from build123d import *

# Parameters (mm, degrees)
ESQUISSE1_W                  = 210
ESQUISSE1_H                  = 90
ESQUISSE1_W_2                = 200
ESQUISSE1_H_2                = 80
BOSS_EXTRU_1_DEPTH           = 5
ESQUISSE2_R                  = 20
ESQUISSE2_R_2                = 15
BOSS_EXTRU_2_DEPTH           = 5
BOSS_EXTRU_3_DEPTH           = 90
BOSS_EXTRU_4_DEPTH           = 200
ESQUISSE6_W                  = 26.875595252
ESQUISSE6_H                  = 32.252188949
ENL_V_MAT_EXTRU_1_DEPTH      = 200
ENL_V_MAT_EXTRU_2_DEPTH      = 200
ENL_V_MAT_EXTRU_3_DEPTH      = 237
ESQUISSE10_R                 = 20
ENL_V_MAT_EXTRU_4_DEPTH      = 6
ENL_V_MAT_EXTRU_4_DEPTH_BACK = 106
ESQUISSE11_W                 = 294.385058415
ESQUISSE11_H                 = 160.265549893
ENL_V_MAT_EXTRU_5_DEPTH      = 23
ENL_V_MAT_EXTRU_5_DEPTH_BACK = 16
BOSS_EXTRU_5_DEPTH           = 5


with BuildPart() as part:
    # Esquisse1 → Boss.-Extru.1 (new body)
    with BuildSketch(Plane.XY):
        with Locations((100, -26.819835627)):
            Rectangle(ESQUISSE1_W, ESQUISSE1_H)
        with Locations((100, -26.819835627)):
            Rectangle(ESQUISSE1_W_2, ESQUISSE1_H_2, mode=Mode.SUBTRACT)
    extrude(amount=BOSS_EXTRU_1_DEPTH)



with BuildPart() as body_2:
    # Esquisse2 → Boss.-Extru.2 (new body)
    with BuildSketch(Plane.XY.offset(105)):
        with Locations((100, -26.819835627)):
            Circle(ESQUISSE2_R)
        with Locations((100, -26.819835627)):
            Circle(ESQUISSE2_R_2, mode=Mode.SUBTRACT)
    extrude(amount=BOSS_EXTRU_2_DEPTH)


with BuildPart() as part_1:
    add(part.part)

    add(body_2.part)  # Boss.-Extru.3 merges body 2
    # Esquisse3 → Boss.-Extru.3 (add)
    with BuildSketch(Plane.XZ.offset(71.819835627)):
        Polygon((113.437797626, 105), (198.437797626, 5), (205, 5), (119.954563332, 105), align=None)
        Polygon((80, 105), (-5, 5), (1.562202374, 5), (86.562202374, 105), align=None)
    extrude(amount=-BOSS_EXTRU_3_DEPTH)

    # Esquisse5 → Boss.-Extru.4 (add)
    with BuildSketch(Plane.ZY.offset(-200)):
        Polygon((5, 18.180164373), (105, -5.554833167), (105, -10.693741152), (5, 13.041256389), align=None)
        Polygon((5, -71.819835627), (105, -48.084838086), (105, -42.945930101), (5, -66.680927642), align=None)
    extrude(amount=BOSS_EXTRU_4_DEPTH)

    # Esquisse6 → Enlèv. mat.-Extru.1 (cut)
    with BuildSketch(Plane(origin=(0, 0, 105), x_dir=(-1, 0, 0), z_dir=(0, 0, -1))):
        with Locations((-100, -26.819835627)):
            Rectangle(ESQUISSE6_W, ESQUISSE6_H)
    extrude(amount=-ENL_V_MAT_EXTRU_1_DEPTH, mode=Mode.SUBTRACT)

    # Esquisse8 → Enlèv. mat.-Extru.2 (cut)
    with BuildSketch(Plane.XZ.offset(71.819835627)):
        Polygon((0, 105), (80, 105), (0, 10.882352941), align=None)
        Polygon((120, 105), (200, 10.882352941), (200, 105), align=None)
    extrude(amount=-ENL_V_MAT_EXTRU_2_DEPTH, mode=Mode.SUBTRACT)

    # Esquisse9 → Enlèv. mat.-Extru.3 (cut)
    with BuildSketch(Plane.ZY.offset(5)):
        Polygon((105, 18.180164373), (105, -5.554833167), (5, 18.180164373), align=None)
        Polygon((5, -71.819835627), (105, -71.819835627), (105, -48.084838086), align=None)
    extrude(amount=-ENL_V_MAT_EXTRU_3_DEPTH, mode=Mode.SUBTRACT)

    # Esquisse10 → Enlèv. mat.-Extru.4 (cut, two sides)
    with BuildSketch(Plane.XY.offset(105)) as enl_v_mat_extru_4_sk:
        with Locations((100, -26.819835627)):
            Circle(ESQUISSE10_R)
    extrude(amount=ENL_V_MAT_EXTRU_4_DEPTH, mode=Mode.SUBTRACT)
    extrude(enl_v_mat_extru_4_sk.sketch, amount=-ENL_V_MAT_EXTRU_4_DEPTH_BACK, mode=Mode.SUBTRACT)

    # Esquisse11 → Enlèv. mat.-Extru.5 (cut, two sides)
    with BuildSketch(Plane(origin=(0, 13.180164373, 0), x_dir=(-1, 0, 0), z_dir=(0, -1, 0))) as enl_v_mat_extru_5_sk:
        with Locations((-99.239876108, -40.996630143)):
            Rectangle(ESQUISSE11_W, ESQUISSE11_H)
    extrude(amount=ENL_V_MAT_EXTRU_5_DEPTH, mode=Mode.SUBTRACT)
    extrude(enl_v_mat_extru_5_sk.sketch, amount=-ENL_V_MAT_EXTRU_5_DEPTH_BACK, mode=Mode.SUBTRACT)

    # Esquisse12 → Boss.-Extru.5 (add)
    with BuildSketch(Plane(origin=(0, -9.819835627, 0), x_dir=(1, 0, 0), z_dir=(0, 1, 0))):
        Polygon((-5, -5), (-5, 0), (205, 0), (205, -5), (120, -105), (80, -105), align=None)
    extrude(amount=BOSS_EXTRU_5_DEPTH)


solid = part_1.part
For this review, take the finished solid that the model builds, in its own axes (mm). A direction names the side the tool comes from. Give positions to 0.01 mm unless a question says otherwise; leave off trailing zeros. Order: outer loops, then holes, each group sorted by start corner. A loop starts at its lowest first (then second) coordinate and runs counter-clockwise, first axis right, second up. Notation, with made-up numbers: (-6.5, 27.25) -> (34.5, 27.25) arc R22 ccw to (34.5, 56.25) -> close; hole circle Ø10 at (-14.5, -31.75). An arc over 180 degrees is marked (long way). Write item = value, one per line.
1) Draft analysis for pull direction Y (two halves, no side actions). For faces 4 (the face through (164.787, -32.331, 44.589)), 5 (the face through (163.095, -7.145, 54.3)), 6 (the face through (99, -71.82, 3)), state which applies: pulls with the +Y half, pulls with the -Y half, needs draft (parallel to the pull), parting line crosses it, or undercut.
Findings:
face_4 = undercut
face_5 = needs draft
face_6 = pulls with the -Y half
2) Insertion check: pin 1 (1.5 mm diameter, centred on y = -12.5, z = 30.5, fed in from -X); pin 2 (1 mm diameter, centred on x = 66, z = 53.5, fed in from -Y); pin 3 (6 mm diameter, centred on x = 35.5, y = -13, fed in from -Z). Each pin has a flat end and moves straight along its axis. Give the tip position at first contact, or say it passes through.
Findings:
pin_1 = 16.04
pin_2 = -60.43
pin_3 = 41.4
3) We need section B-B, the plane z = 47.5. Give the boundary of the cut face in (x, y) (3 decimals), and give its area (3 significant figures).
Findings:
outline = (31.125, -61.732) -> (168.875, -61.732) -> (168.875, -56.594) -> (168.856, -56.594) -> (168.856, -9.82) -> (168.875, -9.82) -> (168.875, -4.82) -> (31.125, -4.82) -> close; hole (37.687, -56.594) -> (162.313, -56.594) -> (162.313, -9.82) -> (37.687, -9.82) -> close
area = 2,010 mm^2
4) To check wall thickness, follow L1, parallel to Z at x = 80, y = -35; L2, parallel to X at y = -44.5, z = 16 (3 decimals); L3, parallel to X at y = -53, z = 52.5 (3 decimals). State the ranges of each line that lie inside material, in increasing order. Write a range as from..to.
Findings:
L1 = 97.28..105
L2 = 4.35..10.912, 189.088..195.645
L3 = 35.375..41.937, 158.063..164.603
5) For faces 1 (the face through (80, -27, 102)), 2 (the face through (86.491, -10.166, 102.776)), 3 (the face through (205, -39, 2)), list the 3-axis set-ups (+Z, -Z, +X, -X, +Y, -Y) from which the entire face can be reached by the end or side of a thin tool; tool diameter is ignored.
Findings:
face_1 = +Z, -Z
face_2 = -Z
face_3 = +Z, -Z, +X, +Y, -Y
6) We need section A-A, the plane y = -35.5. Give the boundary of the cut face in (x, z), and give its area (3 significant figures).
Findings:
outline = (-5, 0) -> (0, 0) -> (0, 5) -> (1.56, 5) -> (81.98, 99.61) -> (81.98, 105) -> (80, 105) -> (-5, 5) -> close; (118.02, 99.61) -> (198.44, 5) -> (200, 5) -> (200, 0) -> (205, 0) -> (205, 5) -> (119.95, 105) -> (118.02, 105) -> close
area = 1,340 mm^2
